from build123d import *

# Parameters (mm, degrees)
SKETCH1_4_R         = 10
SKETCH1_4_W         = 2.5
SKETCH1_4_H         = 20
BOSS_EXTRUDE3_DEPTH = 1.25
SKETCH2_W           = 20
SKETCH2_H           = 2.5
CUT_EXTRUDE1_DEPTH  = 72.632743909


with BuildPart() as part:
    # Sketch1_4 → Boss-Extrude3 (new, symmetric)
    # profile 1 of 3: a face of its own
    with BuildSketch(Plane(origin=(0, 0, 0), x_dir=(0, 0, -1), z_dir=(1, 0, 0))):
        Polygon((-26.666666667, -30), (-26.666666667, -25), (26.666666667, -25), (26.666666667, -30), (46.666666667, -30), (46.666666667, -25), (58.5, -25), (58.5, 25), (46.666666667, 25), (46.666666667, 27.5), (26.666666667, 27.5), (26.666666667, 25), (-26.666666667, 25), (-26.666666667, 27.5), (-46.666666667, 27.5), (-46.666666667, 25), (-58.5, 25), (-58.5, -25), (-46.666666667, -25), (-46.666666667, -30), align=None)
        Circle(SKETCH1_4_R, mode=Mode.SUBTRACT)
    # profile 2 of 3: a face of its own
    with BuildSketch(Plane(origin=(0, 0, 0), x_dir=(0, 0, -1), z_dir=(1, 0, 0))):
        Polygon((-63.333333333, -25), (-58.5, -25), (-58.5, 25), (-63.333333333, 25), (-65, 25), (-65, -25), align=None)
        with Locations((-61.75, 0)):
            Rectangle(SKETCH1_4_W, SKETCH1_4_H, mode=Mode.SUBTRACT)
    # profile 3 of 3: a face of its own
    with BuildSketch(Plane(origin=(0, 0, 0), x_dir=(0, 0, -1), z_dir=(1, 0, 0))):
        Polygon((58.5, 25), (58.5, -25), (63.333333333, -25), (65, -25), (65, 25), (63.333333333, 25), align=None)
        with Locations((61.75, 0)):
            Rectangle(SKETCH1_4_W, SKETCH1_4_H, mode=Mode.SUBTRACT)
    extrude(amount=BOSS_EXTRUDE3_DEPTH, both=True)

    # Sketch2 → Cut-Extrude1 (cut, through all)
    with BuildSketch(Plane(origin=(1.25, 0, 0), x_dir=(0, 0, -1), z_dir=(1, 0, 0))):
        with Locations((-36.666666667, 18.75)):
            Rectangle(SKETCH2_W, SKETCH2_H)
        with Locations((-36.666666667, 11.25)):
            Rectangle(SKETCH2_W, SKETCH2_H)
        with Locations((-36.666666667, 3.75)):
            Rectangle(SKETCH2_W, SKETCH2_H)
        with Locations((-36.666666667, -3.75)):
            Rectangle(SKETCH2_W, SKETCH2_H)
        with Locations((-36.666666667, -11.25)):
            Rectangle(SKETCH2_W, SKETCH2_H)
        with Locations((-36.666666667, -18.75)):
            Rectangle(SKETCH2_W, SKETCH2_H)
        with Locations((36.666666667, -18.75)):
            Rectangle(SKETCH2_W, SKETCH2_H)
        with Locations((36.666666667, -11.25)):
            Rectangle(SKETCH2_W, SKETCH2_H)
        with Locations((36.666666667, -3.75)):
            Rectangle(SKETCH2_W, SKETCH2_H)
        with Locations((36.666666667, 3.75)):
            Rectangle(SKETCH2_W, SKETCH2_H)
        with Locations((36.666666667, 11.25)):
            Rectangle(SKETCH2_W, SKETCH2_H)
        with Locations((36.666666667, 18.75)):
            Rectangle(SKETCH2_W, SKETCH2_H)
    extrude(amount=-CUT_EXTRUDE1_DEPTH, mode=Mode.SUBTRACT)


solid = part.part
For this review, take the finished solid that the model builds, in its own axes (mm). A direction names the side the tool comes from. Coordinates: 2 decimals unless noted, no trailing zeros. Loops run counter-clockwise (first coordinate to the right, second up) from the corner with the lowest first, then second, coordinate; pieces in that order, holes last. Notation, with made-up numbers: (80, 59) - (128, 59) arc R23 cw to (128, 98) - close; hole circle Ø3 at (42, 0.5). An arc over 180 degrees is marked (long way). Return JSON: item names as keys, results as strings.
Item 1: Mouldability with a two-part tool opening along Z and no side actions: class faces 1 (the flat face through (0, 26, -46.667)), 2 (the flat face through (0, 27.5, 37)), 3 (the flat face through (0, 5, -37)) as pulls with the +Z half, pulls with the -Z half, needs draft (parallel to the pull), parting line crosses it, or undercut.
Determined:
{"face 1": "pulls with the -Z half", "face 2": "needs draft", "face 3": "undercut"}
Item 2: Take a section at B-B (y = 0). Give the boundary of the cut face in (x, z), then the cut area to 4 significant figures.
Determined:
{"outline": "(-1.25, -65) - (1.25, -65) - (1.25, -63) - (-1.25, -63) - close; (-1.25, -60.5) - (1.25, -60.5) - (1.25, -10) - (-1.25, -10) - close; (-1.25, 10) - (1.25, 10) - (1.25, 60.5) - (-1.25, 60.5) - close; (-1.25, 63) - (1.25, 63) - (1.25, 65) - (-1.25, 65) - close", "area": "262.5 mm2"}
Item 3: Take a section at A-A (z = 0). Give the boundary of the cut face in (x, y), then the cut area to 3 significant figures.
Determined:
{"outline": "(-1.25, -25) - (1.25, -25) - (1.25, -10) - (-1.25, -10) - close; (-1.25, 10) - (1.25, 10) - (1.25, 25) - (-1.25, 25) - close", "area": "75.0 mm2"}
Item 4: For line 1 (Z direction, x = 0.65, y = -12); line 2 (Z direction, x = 0.1, y = 0.5); line 3 (Z direction, x = -1, y = 8), list the stretches that pass through material, from the lowest coordinate up.
Determined:
{"line 1": "z = -65 to -46.67, -26.67 to 26.67, 46.67 to 65", "line 2": "z = -65 to -63, -60.5 to -9.99, 9.99 to 60.5, 63 to 65", "line 3": "z = -65 to -63, -60.5 to -6, 6 to 60.5, 63 to 65"}
Item 5: For faces 4 (the flat face through (0, -4, -26.667)), 5 (the flat face through (0, 26, 46.667)), 6 (the flat face through (0, -28, -46.667)), 7 (the flat face through (0, 0, 65)), list the 3-axis set-ups (+Z, -Z, +X, -X, +Y, -Y) from which the entire face can be reached by the end or side of a thin tool; tool diameter is ignored.
Determined:
{"face 4": "+X, -X", "face 5": "+Z, +X, -X, +Y", "face 6": "-Z, +X, -X, -Y", "face 7": "+Z, +X, -X, +Y, -Y"}
Item 6: Take a section at C-C (x = -0.6). State how many separate pieces and enclosed holes the cut face has, then the cut area to 3 significant figures.
Determined:
{"separate pieces": "1", "enclosed holes": "15", "area": "5,790 mm2"}
Item 7: Take a section at D-D (z = -48). Give the boundary of the cut face in (x, y), then the cut area to 3 significant figures.
Determined:
{"outline": "(-1.25, -25) - (1.25, -25) - (1.25, 25) - (-1.25, 25) - close", "area": "125 mm2"}
